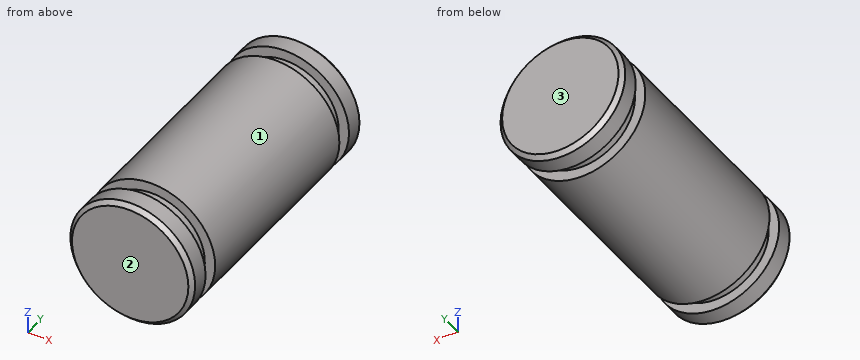
```python
from build123d import *

# Parameters (mm, degrees)
SKETCH1_W       = 3
SKETCH1_H       = 13
SKETCH5_W       = 2.05
SKETCH5_H       = 0.74
CHANFREIN1_SIZE = 0.2


with BuildPart() as part:
    # Sketch1 → Revolve1 (revolve)
    with BuildSketch(Plane.XY):
        with Locations((1.5, 6.5)):
            Rectangle(SKETCH1_W, SKETCH1_H)
    revolve(axis=Axis((0, 0, 0), (0, 1, 0)))

    # Sketch5 → Groove for DIN 471 - 4 x 0.4, Circlip for shafts - normal1 (revolve, cut)
    with BuildSketch(Plane(origin=(0, 0, 0), x_dir=(0, 0, -1), z_dir=(-1, 0, 0))):
        with Locations((3.525, -1.37)):
            Rectangle(SKETCH5_W, SKETCH5_H)
        with Locations((3.525, -11.63)):
            Rectangle(SKETCH5_W, SKETCH5_H)
    revolve(axis=Axis((0, 50.028808754, 0), (0, -1, 0)), mode=Mode.SUBTRACT)

    # Chanfrein1
    chanfrein1_edges = [part.edges().sort_by_distance(p)[0] for p in [
        (-3, 0, 0),
        (-3, 13, 0),
    ]]
    chamfer(chanfrein1_edges, length=CHANFREIN1_SIZE)


solid = part.part
```
Model file for the job. Use its own axes, mm. Face numbers are marked on the shaded views. Give positions to 0.01 mm unless a question says otherwise; leave off trailing zeros. Write each loop counter-clockwise with the first axis right and the second up, starting at its lowest first coordinate (ties: lowest second). Pieces come first, ordered by that corner, then holes. Notation, with made-up numbers: (62.5, -2.5) - (75.5, -2.5) arc R17 cw to (75.5, 18.5) - close; hole circle Ø10 at (-14, 48). An arc over 180 degrees is marked (long way). One line per question, with ' | ' between items. Start each with the question number.
(1) Slice it at B-B on x = 0. Write the cut outline in (y, z).
(2) Pin check, flat tip, straight feed: P1, Ø3, axis at x = 1.5, z = 0.5, coming from the -Y side. Stop position of the tip, or through.
(3) Wall check: line 1 along Y through (x, z) = (-2.5, 0.7); line 2 along Z through (x, y) = (-0.1, 0.5); line 3 along X through (y, z) = (2.5, 2.2). Give the ranges that are in metal, low to high. Write a range as from..to.
(4) Slice it at A-A on z = 0. Write the cut outline in (x, y).
(5) Slice it at C-C on y = 8.75. Write the cut outline in (x, z), plus the area to 3 significant figures.
(6) Two-plate mould, pull along Y, no slides. Class the marked faces 1, 2 and 3: +Y half, -Y half, draft (parallel to the pull), parting line (faces both ways), or undercut.
Results below:
1) outline: (0, -2.8) - (0.2, -3) - (1, -3) - (1, -2.5) - (1.74, -2.5) - (1.74, -3) - (11.26, -3) - (11.26, -2.5) - (12, -2.5) - (12, -3) - (12.8, -3) - (13, -2.8) - (13, 2.8) - (12.8, 3) - (12, 3) - (12, 2.5) - (11.26, 2.5) - (11.26, 3) - (1.74, 3) - (1.74, 2.5) - (1, 2.5) - (1, 3) - (0.2, 3) - (0, 2.8) - close
2) P1: y = 0
3) line 1: 0..1, 1.74..11.26, 12..13 | line 2: -3..3 | line 3: -2.04..2.04
4) outline: (-3, 0.2) - (-2.8, 0) - (2.8, 0) - (3, 0.2) - (3, 1) - (2.5, 1) - (2.5, 1.74) - (3, 1.74) - (3, 11.26) - (2.5, 11.26) - (2.5, 12) - (3, 12) - (3, 12.8) - (2.8, 13) - (-2.8, 13) - (-3, 12.8) - (-3, 12) - (-2.5, 12) - (-2.5, 11.26) - (-3, 11.26) - (-3, 1.74) - (-2.5, 1.74) - (-2.5, 1) - (-3, 1) - close
5) outline: circle Ø6 at (0, 0) | area: 28.3 mm^2
6) face 1: draft | face 2: -Y half | face 3: +Y half
